from build123d import *

# Parameters (mm, degrees)
F0_W         = 69.85
F0_H         = 19.05
F1_DEPTH     = 19.05
F2_R         = 11.90625
F3_DEPTH     = 12.7
F4_R         = 7.9375
F5_DEPTH     = 9.525
F6_W         = 38.1
F6_H         = 12.7
F7_DEPTH     = 12.7
F8_R         = 2.38125
F9_DEPTH     = 25.4
F10_R        = 8.6959968999
F11_DEPTH    = 69.851
F12_R        = 1.5875
F13_C1_SIZE2 = 9.525
F13_C1_SIZE  = 22.225
F13_C2_SIZE2 = 22.225
F13_C2_SIZE  = 9.525


# Not quite as in the source:
# - two fillets or chamfers of one size are made in one step


with BuildPart() as f1:
    # F0 (on Top) → F1 (new body)
    with BuildSketch(Plane.XY):
        with Locations((34.925, 9.525)):
            Rectangle(F0_W, F0_H)
    extrude(amount=F1_DEPTH)

    # F2 (on face) → F3 (cut)
    with BuildSketch(Plane.XY.offset(19.05)):
        with Locations((34.925, 9.525)):
            Circle(F2_R)
    extrude(amount=-F3_DEPTH, mode=Mode.SUBTRACT)

    # F4 (on face) → F5 (join)
    with BuildSketch(Plane.XY.offset(6.35)):
        with Locations((34.925, 9.525)):
            Circle(F4_R)
    extrude(amount=F5_DEPTH)

    # F6 (on face) → F7 (cut)
    with BuildSketch(Plane.XY.offset(19.05)):
        with Locations((69.85, 9.525)):
            Rectangle(F6_W, F6_H)
        with Locations((0, 9.525)):
            Rectangle(F6_W, F6_H)
    extrude(amount=-F7_DEPTH, mode=Mode.SUBTRACT)

    # F8 (on face) → F9 (cut)
    with BuildSketch(Plane.XY.offset(6.35)):
        with Locations((63.5, 9.525)):
            Circle(F8_R)
        with Locations((6.35, 9.5145329833)):
            Circle(F8_R)
    extrude(amount=-F9_DEPTH, mode=Mode.SUBTRACT)

    # F10 (on face) → F11 (cut, through all)
    with BuildSketch(Plane.YZ.offset(69.85)):
        with Locations((9.525, -4.7272468999)):
            Circle(F10_R)
    extrude(amount=-F11_DEPTH, mode=Mode.SUBTRACT)

    # F12
    f12_edges = [f1.edges().sort_by_distance(p)[0] for p in [
        (26.9875, 9.525, 15.875),
    ]]
    fillet(f12_edges, radius=F12_R)

    # F13: chamfer of 9.525 x 22.225 on 4 edges, made by hand

    # F13_c1
    f13_c1_edges = [f1.edges().sort_by_distance(p)[0] for p in [
        (69.85, 17.4625, 19.05),
    ]]
    f13_c1_side = f1.faces().sort_by_distance((69.6595, 17.4625, 19.05))[0]
    chamfer(f13_c1_edges, length=F13_C1_SIZE, length2=F13_C1_SIZE2, reference=f13_c1_side)

    # F13_c2
    f13_c2_edges = [f1.edges().sort_by_distance(p)[0] for p in [
        (0, 1.5875, 19.05),
    ]]
    f13_c2_side = f1.faces().sort_by_distance((0, 1.5875, 18.8595))[0]
    chamfer(f13_c2_edges, length=F13_C2_SIZE, length2=F13_C2_SIZE2, reference=f13_c2_side)


solid = f1.part
Read the model definition and answer for the solid it produces. Units are mm, in the model's axes. A direction names the side the tool comes from. Give positions to 0.01 mm unless a question says otherwise; leave off trailing zeros. Write each loop counter-clockwise with the first axis right and the second up, starting at its lowest first coordinate (ties: lowest second). Pieces come first, ordered by that corner, then holes. Notation, with made-up numbers: M 84.5,36.25 L 143.5,36.25 A16 cw 143.5,40.25 Z; hole C 36,36.5 d5. An arc over 180 degrees is marked long. One line per item, written item: value. Start each with the question number.
(1) Find section A-A (z = 12). Give the number of separate pieces and of enclosed holes in the cut face, plus the area to 3 significant figures.
(2) Determine the mould class of faces 5 (the flat face through (0, 9, 5)), 6 (the flat face through (26.8, 9.7, 6.35)) for opening direction Y: pulls with the +Y half, pulls with the -Y half, needs draft (parallel to the pull), parting line crosses it, or undercut.
(3) Find the intervals of material crossed by line 1 (Y direction, x = 54, z = 11.5) (3 decimals); line 2 (X direction, y = 13.75, z = 6.75); line 3 (Y direction, x = 63.5, z = 5.4), in increasing order.
(4) A tool of negligible diameter and unlimited length cuts with its end or side. For faces 1 (the cylindrical face through (8.55, 8.6, 5.01)), 2 (the flat face through (58, 15.875, 11)), 3 (the flat face through (9, 10, 6.35)), 4 (the cylindrical face through (46.83, 9.37, 12.79)), from which of +Z, -Z, +X, -X, +Y, -Y can it reach the whole face along a straight path? Write none if from no direction.
(5) Find section B-B (x = 6.35). Determine the outline of the cut face in (y, z) (3 decimals).
(6) Find section C-C (x = 56.5). Determine the outline of the cut face in (y, z) (3 decimals).
(7) Find section D-D (x = 25). Determine the outline of the cut face in (y, z) (3 decimals).
(8) Flat-ended cylindrical pins translate along their axes: pin 1 Ø5.5 at (x, y) = (6.35, 9.51) entering from -Z; pin 2 Ø5 at (x, z) = (31, 9.5) entering from +Y; pin 3 Ø10 at (x, z) = (11.5, 16) entering from +Y; pin 4 Ø4 at (x, y) = (32, 10) entering from +Z (3 decimals). Find the tip coordinate at first contact, or state that the pin passes through.
Results below:
1. separate pieces: 3
1. enclosed holes: 0
1. area: 572 mm^2
2. face 5: needs draft
2. face 6: undercut
3. line 1: y = 0 to 3.175, 15.875 to 19.05
3. line 2: x = 19.05 to 23.79, 28.21 to 41.64, 46.06 to 50.8
3. line 3: y = 0 to 7.14, 11.91 to 19.05
4. face 1: +Z, -Z
4. face 2: +Z, +X
4. face 3: +Z, -X
4. face 4: +Z
5. outline: M 0,0 L 2.226,0 A8.696 cw 7.133,3.633 L 7.133,6.35 L 3.175,6.35 L 3.175,12.246 L 0,12.246 Z; M 11.896,3.639 A8.696 cw 16.824,0 L 19.05,0 L 19.05,12.246 L 15.875,12.246 L 15.875,6.35 L 11.896,6.35 Z
6. outline: M 0,0 L 2.226,0 A8.696 cw 16.824,0 L 19.05,0 L 19.05,15.246 L 15.875,15.246 L 15.875,6.35 L 3.175,6.35 L 3.175,15.246 L 0,15.246 Z
7. outline: M 0,0 L 2.226,0 A8.696 cw 16.824,0 L 19.05,0 L 19.05,19.05 L 16.102,19.05 L 16.102,6.35 L 2.948,6.35 L 2.948,19.05 L 0,19.05 Z
8. pin 1: stops at z = 3.52
8. pin 2: stops at y = 17.33
8. pin 3: stops at y = 19.05
8. pin 4: stops at z = 15.875
